Check sheet for the modelled part. Datum: model origin and axes. Units: mm. A direction names the side the tool comes from. Give positions to 0.01 mm unless a question says otherwise; leave off trailing zeros. Order: outer loops, then holes, each group sorted by start corner. A loop starts at its lowest first (then second) coordinate and runs counter-clockwise, first axis right, second up. Notation, with made-up numbers: (-26.5, 76.5) -> (-7.5, 76.5) arc R24 cw to (-7.5, 94.5) -> close; hole circle Ø4 at (89, 2). An arc over 180 degrees is marked (long way). Answer in a Markdown table with one row per item. Add a question column.
(1) Cross-section at A-A (x = 0). Record the cut outline in (y, z).
(2) Go/stop test with flat-tipped pins: pin 1 (5 mm diameter, centred on x = 0, y = 0, fed in from +Z); pin 2 (4 mm diameter, centred on x = 1.5, y = -6.5, fed in from -Z); pin 3 (1 mm diameter, centred on y = -2.5, z = 2, fed in from -X); pin 4 (3 mm diameter, centred on y = -8.5, z = 3.5, fed in from +X). Record where each tip stops, or that it passes through.
(3) Cross-section at C-C (z = 8). Record the cut outline in (x, y).
(4) Thickness scan on L1, parallel to Y at x = 0, z = 4.75; L2, parallel to Z at x = -0.25, y = 9; L3, parallel to Y at x = 1.5, z = 11.75. Record the ranges inside material, lowest first. Write a range as [from, to].
(5) Set-up check for faces 4 (the face through (-1.4, 10.66, 1.73)), 5 (the face through (2, -5, 3.5)): record each of +Z, -Z, +X, -X, +Y, -Y from which the full face is reachable in a straight line by a thin tool's end or side.
(6) Cross-section at D-D (x = -8.75). Record the cut outline in (y, z) (3 decimals).
(7) Release check for a two-part mould opening along Y. For faces 1 (the face through (-1.08, -4.88, 8.43)), 2 (the face through (-0.867, -3.905, 6.844)), 3 (the face through (5, 0, 0)) record: released by +Y, released by -Y, zero draft, split by the parting line, or undercut.
```python
from build123d import *

# Parameters (mm, degrees)
SKETCH1_R           = 10.75
BOSS_EXTRUDE1_DEPTH = 3.5
SKETCH2_R           = 5
BOSS_EXTRUDE2_DEPTH = 10
CUT_EXTRUDE1_REACH  = 22.332
SKETCH3_R           = 4


with BuildPart() as part:
    # Sketch1 → Boss-Extrude1 (new body)
    with BuildSketch(Plane.XY):
        Circle(SKETCH1_R)
    extrude(amount=BOSS_EXTRUDE1_DEPTH)

    # Sketch2 → Boss-Extrude2 (add)
    with BuildSketch(Plane.XY.offset(3.5)):
        Circle(SKETCH2_R)
    extrude(amount=BOSS_EXTRUDE2_DEPTH)

    # Sketch3 → Cut-Extrude1 (cut, up to next)
    with BuildSketch(Plane.XY.offset(13.5), mode=Mode.PRIVATE) as cut_extrude1_sk1:
        Circle(SKETCH3_R)
    cut_extrude1_tool1 = extrude(cut_extrude1_sk1.sketch, amount=-CUT_EXTRUDE1_REACH, mode=Mode.PRIVATE) & part.part
    add(cut_extrude1_tool1.solids().sort_by_distance((0, 0, 13.5))[0], mode=Mode.SUBTRACT)


solid = part.part
```
Answer below:
| question | item | result |
|---|---|---|
| 1 | outline | (-10.75, 0) -> (-4, 0) -> (-4, 13.5) -> (-5, 13.5) -> (-5, 3.5) -> (-10.75, 3.5) -> close; (4, 0) -> (10.75, 0) -> (10.75, 3.5) -> (5, 3.5) -> (5, 13.5) -> (4, 13.5) -> close |
| 2 | pin 1 | passes through |
| 2 | pin 2 | stops at z = 0 |
| 2 | pin 3 | stops at x = -10.56 |
| 2 | pin 4 | stops at x = 8.16 |
| 3 | outline | circle Ø10 at (0, 0); hole circle Ø8 at (0, 0) |
| 4 | L1 | y = [-5, -4], [4, 5] |
| 4 | L2 | z = [0, 3.5] |
| 4 | L3 | y = [-4.77, -3.71], [3.71, 4.77] |
| 5 | face 4 | +Z, -Z |
| 5 | face 5 | +Z |
| 6 | outline | (-6.245, 0) -> (6.245, 0) -> (6.245, 3.5) -> (-6.245, 3.5) -> close |
| 7 | face 1 | split by the parting line |
| 7 | face 2 | undercut |
| 7 | face 3 | zero draft |
